from build123d import *

# Parameters (mm, degrees)
SKETCH1_W               = 46.5
SKETCH1_H               = 24
BOSS_EXTRUDE1_DEPTH     = 21
SHELL1_T                = -1.25
SKETCH2_W               = 19.75
SKETCH2_H               = 14.5
CUT_EXTRUDE1_DEPTH      = 47.5
SKETCH7_W               = 10.375
SKETCH7_H               = 2.5
CUT_EXTRUDE5_DEPTH      = 1.25
SKETCH9_W               = 19.5
SKETCH9_H               = 6
BOSS_EXTRUDE3_DEPTH     = 2.5
CUT_EXTRUDE7_START      = -45.25
SKETCH12_W              = 1.5
SKETCH12_H              = 8.25
CUT_EXTRUDE7_DEPTH      = 46.25
CUT_EXTRUDE7_DEPTH_BACK = 47.5
SKETCH13_W              = 2.75
SKETCH13_H              = 8.25
BOSS_EXTRUDE4_DEPTH     = 44
SKETCH15_W              = 10
SKETCH15_H              = 2.75
BOSS_EXTRUDE5_DEPTH     = 0.75
CUT_EXTRUDE8_REACH      = 23
SKETCH18_W              = 6.76
SKETCH18_H              = 5
CUT_EXTRUDE9_REACH      = 23
SKETCH22_W              = 8.593751287
SKETCH22_H              = 16.011767213
CUT_EXTRUDE15_REACH     = 23
SKETCH25_W              = 10
SKETCH25_H              = 4.5
CUT_EXTRUDE16_REACH     = 26
SKETCH6_R               = 1.9


with BuildPart() as part:
    # Sketch1 → Boss-Extrude1 (new body)
    with BuildSketch(Plane.XY):
        with Locations((22, 12)):
            Rectangle(SKETCH1_W, SKETCH1_H)
    extrude(amount=-BOSS_EXTRUDE1_DEPTH)

    # Shell1
    shell1_openings = [part.faces().sort_by_distance(p)[0] for p in [
        (22, 12, -21),
        (22, 24, -10.5),
    ]]
    offset(amount=SHELL1_T, openings=shell1_openings, kind=Kind.INTERSECTION)

    # Sketch2 → Cut-Extrude1 (cut, through all)
    with BuildSketch(Plane.ZY.offset(1.25)):
        with Locations((-11.125, 8.5)):
            Rectangle(SKETCH2_W, SKETCH2_H)
    extrude(amount=-CUT_EXTRUDE1_DEPTH, mode=Mode.SUBTRACT)

    # Sketch7 → Cut-Extrude5 (cut)
    with BuildSketch(Plane.XY):
        with Locations((40.0625, 2.5)):
            Rectangle(SKETCH7_W, SKETCH7_H)
        with Locations((3.9375, 2.5)):
            Rectangle(SKETCH7_W, SKETCH7_H)
    extrude(amount=-CUT_EXTRUDE5_DEPTH, mode=Mode.SUBTRACT)

    # Sketch9 → Boss-Extrude3 (add)
    with BuildSketch(Plane(origin=(0, 1.25, 0), x_dir=(1, 0, 0), z_dir=(0, 1, 0))):
        with Locations((25.125, 18)):
            Rectangle(SKETCH9_W, SKETCH9_H)
    extrude(amount=BOSS_EXTRUDE3_DEPTH)

    # Sketch12 → Cut-Extrude7 (cut, two sides)
    with BuildSketch(Plane(origin=(45.25, 0, 0), x_dir=(0, 0, -1), z_dir=(1, 0, 0)).offset(CUT_EXTRUDE7_START)) as cut_extrude7_sk:
        with Locations((20.25, 19.875)):
            Rectangle(SKETCH12_W, SKETCH12_H)
    extrude(amount=CUT_EXTRUDE7_DEPTH, mode=Mode.SUBTRACT)
    extrude(cut_extrude7_sk.sketch, amount=-CUT_EXTRUDE7_DEPTH_BACK, mode=Mode.SUBTRACT)

    # Sketch13 → Boss-Extrude4 (add)
    with BuildSketch(Plane(origin=(0, 0, 0), x_dir=(0, 0, -1), z_dir=(1, 0, 0))):
        with Locations((18.125, 19.875)):
            Rectangle(SKETCH13_W, SKETCH13_H)
    extrude(amount=BOSS_EXTRUDE4_DEPTH)

    # Sketch15 → Boss-Extrude5 (add)
    with BuildSketch(Plane.XZ.offset(-15.75)):
        with Locations((29.875, -18.125)):
            Rectangle(SKETCH15_W, SKETCH15_H)
    extrude(amount=BOSS_EXTRUDE5_DEPTH)

    # Sketch18 → Cut-Extrude8 (cut, up to next)
    with BuildSketch(Plane.XY, mode=Mode.PRIVATE) as cut_extrude8_sk1:
        with Locations((10.08, 10.69)):
            Rectangle(SKETCH18_W, SKETCH18_H)
    cut_extrude8_tool1 = extrude(cut_extrude8_sk1.sketch, amount=-CUT_EXTRUDE8_REACH, mode=Mode.PRIVATE) & part.part
    add(cut_extrude8_tool1.solids().sort_by_distance((10.08, 10.69, 0))[0], mode=Mode.SUBTRACT)

    # Sketch22 → Cut-Extrude9 (cut, up to next)
    with BuildSketch(Plane.XY, mode=Mode.PRIVATE) as cut_extrude9_sk1:
        with Locations((21.422492142, 15.994116394)):
            Rectangle(SKETCH22_W, SKETCH22_H)
    cut_extrude9_tool1 = extrude(cut_extrude9_sk1.sketch, amount=-CUT_EXTRUDE9_REACH, mode=Mode.PRIVATE) & part.part
    add(cut_extrude9_tool1.solids().sort_by_distance((21.422492, 15.994116, 0))[0], mode=Mode.SUBTRACT)

    # Sketch25 → Cut-Extrude15 (cut, up to next)
    with BuildSketch(Plane.XY, mode=Mode.PRIVATE) as cut_extrude15_sk1:
        Polygon((31.35, 18.75), (41.85, 18.75), (41.85, 24), (41.6, 24), (41.6, 19.5), (31.6, 19.5), (31.6, 24), (31.35, 24), align=None)
    cut_extrude15_tool1 = extrude(cut_extrude15_sk1.sketch, amount=-CUT_EXTRUDE15_REACH, mode=Mode.PRIVATE) & part.part
    add(cut_extrude15_tool1.solids().sort_by_distance((31.475, 23.882606, 0))[0], mode=Mode.SUBTRACT)
    # Sketch25 → Cut-Extrude15 (cut, up to next)
    with BuildSketch(Plane.XY, mode=Mode.PRIVATE) as cut_extrude15_sk2:
        with Locations((36.6, 21.75)):
            Rectangle(SKETCH25_W, SKETCH25_H)
    cut_extrude15_tool2 = extrude(cut_extrude15_sk2.sketch, amount=-CUT_EXTRUDE15_REACH, mode=Mode.PRIVATE) & part.part
    add(cut_extrude15_tool2.solids().sort_by_distance((36.6, 21.75, 0))[0], mode=Mode.SUBTRACT)

    # Sketch6 → Cut-Extrude16 (cut, up to next)
    with BuildSketch(Plane(origin=(0, 0, 0), x_dir=(-1, 0, 0), z_dir=(0, -1, 0)), mode=Mode.PRIVATE) as cut_extrude16_sk1:
        with Locations((-5.8, 10.25)):
            Circle(SKETCH6_R)
    cut_extrude16_tool1 = extrude(cut_extrude16_sk1.sketch, amount=-CUT_EXTRUDE16_REACH, mode=Mode.PRIVATE) & part.part
    add(cut_extrude16_tool1.solids().sort_by_distance((5.8, 0, -10.25))[0], mode=Mode.SUBTRACT)
    # Sketch6 → Cut-Extrude16 (cut, up to next)
    with BuildSketch(Plane(origin=(0, 0, 0), x_dir=(-1, 0, 0), z_dir=(0, -1, 0)), mode=Mode.PRIVATE) as cut_extrude16_sk2:
        with Locations((-38.2, 10.25)):
            Circle(SKETCH6_R)
    cut_extrude16_tool2 = extrude(cut_extrude16_sk2.sketch, amount=-CUT_EXTRUDE16_REACH, mode=Mode.PRIVATE) & part.part
    add(cut_extrude16_tool2.solids().sort_by_distance((38.2, 0, -10.25))[0], mode=Mode.SUBTRACT)


solid = part.part
Here's how the part is built. I have some questions about the finished solid (model axes, mm). A direction names the side the tool comes from. Round coordinates to 2 decimals unless told otherwise and drop trailing zeros. Write each loop counter-clockwise with the first axis right and the second up, starting at its lowest first coordinate (ties: lowest second). Pieces come first, ordered by that corner, then holes.
1. For faces 1 (the flat face through (0, 20, -9)), 2 (the flat face through (15.375, 2, -18)), 3 (the flat face through (25, 2, -15)), which set-ups out of +Z, -Z, +X, -X, +Y, -Y let a thin tool reach every point of the face, with its end or its side?
2. Suppose I cut it at A-A (x = 38.2). List the corners of the cut face in (y, z) for me.
3. I need wall thicknesses on L1, parallel to X at y = 0.8, z = -10.25; L2, parallel to Y at x = 2.5, z = -18.25; L3, parallel to Z at x = 10, y = 20.5. Which ranges of each line are inside material? Lowest first, please.
4. Suppose I cut it at D-D (z = -10.25). List the corners of the cut face in (x, y) for me.
5. Suppose I cut it at B-B (z = -6). List the corners of the cut face in (x, y) for me.
6. If we mould it in two halves opening along Y, with no side actions, what happens to faces 4 (the flat face through (21, 7.988, -1)), 5 (the flat face through (25.719, 16, -1)), 6 (the flat face through (9, 15.75, -17))? For each: released by +Y, released by -Y, zero draft, split by the parting line, or undercut.
7. Will these pins go through, and if not, where does the flat tip stop? pin 1 Ø1 at (x, z) = (34, -0.5) entering from +Y; pin 2 Ø2 at (y, z) = (4.5, -17.5) entering from -X (3 decimals); pin 3 Ø1.5 at (x, z) = (8.5, -11.5) entering from +Y.
8. Suppose I cut it at C-C (x = 14.5). List the corners of the cut face in (y, z) for me.
Answer sheet:
1. face 1: +Y
1. face 2: -Z, -X
1. face 3: +X, -X, +Y
2. outline: (0, -21) - (1.25, -21) - (1.25, -12.15) - (0, -12.15) - close; (0, -8.35) - (1.25, -8.35) - (1.25, 0) - (0, 0) - close; (3.75, -1.25) - (18.75, -1.25) - (18.75, 0) - (3.75, 0) - close; (15.75, -19.5) - (24, -19.5) - (24, -16.75) - (15.75, -16.75) - close
3. L1: x = -1.25 to 3.9, 7.7 to 36.3, 40.1 to 45.25
3. L2: y = 0 to 1.25, 15.75 to 24
3. L3: z = -19.5 to -16.75, -1.25 to 0
4. outline: (-1.25, 0) - (3.9, 0) - (3.9, 1.25) - (-1.25, 1.25) - close; (-1.25, 15.75) - (0, 15.75) - (0, 24) - (-1.25, 24) - close; (7.7, 0) - (36.3, 0) - (36.3, 1.25) - (7.7, 1.25) - close; (40.1, 0) - (45.25, 0) - (45.25, 1.25) - (40.1, 1.25) - close; (44, 15.75) - (45.25, 15.75) - (45.25, 24) - (44, 24) - close
5. outline: (-1.25, 0) - (45.25, 0) - (45.25, 1.25) - (-1.25, 1.25) - close; (-1.25, 15.75) - (0, 15.75) - (0, 24) - (-1.25, 24) - close; (44, 15.75) - (45.25, 15.75) - (45.25, 24) - (44, 24) - close
6. face 4: released by +Y
6. face 5: zero draft
6. face 6: undercut
7. pin 1: stops at y = 18.75
7. pin 2: stops at x = 15.375
7. pin 3: stops at y = 1.25
8. outline: (0, -21) - (1.25, -21) - (1.25, -1.25) - (24, -1.25) - (24, 0) - (0, 0) - close; (15.75, -19.5) - (24, -19.5) - (24, -16.75) - (15.75, -16.75) - close
